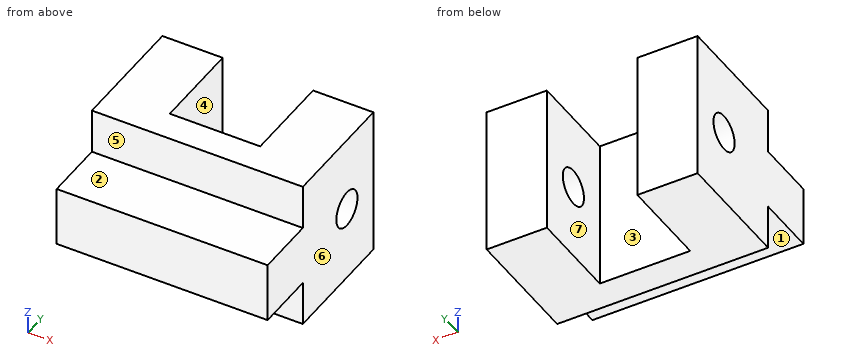
from build123d import *

# Parameters (mm, degrees)
BOSS_EXTRUDE1_DEPTH = 25
SKETCH4_R           = 3
CUT_EXTRUDE1_DEPTH  = 40
SKETCH5_W           = 35
SKETCH5_H           = 10
BOSS_EXTRUDE3_DEPTH = 10


with BuildPart() as part:
    # Sketch1 → Boss-Extrude1 (new body)
    with BuildSketch(Plane.XY):
        Polygon((0, 9.105075836), (0, -5.894924164), (-15, -5.894924164), (-15, 9.105075836), (-25, 9.105075836), (-25, -10.894924164), (10, -10.894924164), (10, 9.105075836), align=None)
    extrude(amount=-BOSS_EXTRUDE1_DEPTH)

    # Sketch4 → Cut-Extrude1 (cut)
    with BuildSketch(Plane(origin=(10, 0, 0), x_dir=(0, 0, -1), z_dir=(1, 0, 0))):
        with Locations(Location((12.5, 1.605075836, 0), (0, 0, 90))):
            Circle(SKETCH4_R)
    extrude(amount=-CUT_EXTRUDE1_DEPTH, mode=Mode.SUBTRACT)

    # Sketch5 → Boss-Extrude3 (add)
    with BuildSketch(Plane.XZ.offset(10.894924164)):
        with Locations((-7.5, -12.5)):
            Rectangle(SKETCH5_W, SKETCH5_H)
    extrude(amount=BOSS_EXTRUDE3_DEPTH)


solid = part.part
CAD build for the part. Positions are in the model's coordinates, mm. Face numbers are marked on the shaded views. A direction names the side the tool comes from. Give positions to 0.01 mm unless a question says otherwise; leave off trailing zeros. Loops run counter-clockwise (first coordinate to the right, second up) from the corner with the lowest first, then second, coordinate; pieces in that order, holes last. Notation, with made-up numbers: M -10.75,3.5 L -2.75,3.5 A18 cw -2.75,9.5 Z; hole C 50,0.5 d9. An arc over 180 degrees is marked long. Answer in a Markdown table with one row per item. Add a question column.
Item 1: Band-saw the part on A-A on y = 7. Give the cut face in (x, z), then the cut area to 3 significant figures.
Item 2: Drop flat-ended pins along their axis: P1, Ø5, axis at x = -14.5, y = -15.5, coming from the -Z side; P2, Ø11, axis at x = -4, y = -16, coming from the +Z side; P3, Ø2, axis at x = -19.5, z = -19, coming from the -Y side; P4, Ø1.5, axis at x = -10, y = -13.5, coming from the +Z side. Give the stop position or say it passes through.
Item 3: Probe probe 1 along X at (y, z) = (-5.5, -6.25); probe 2 along Z at (x, y) = (-1, -17); probe 3 along Z at (x, y) = (-18.5, 0). List the from-to ranges inside material, lowest first.
Item 4: Band-saw the part on D-D on x = -14. Give the cut face in (y, z), then the cut area to 3 significant figures.
Item 5: Mould opens along X. For the marked faces 4, 5, 6 and 7 say: +X half, -X half, draft (parallel to the pull), parting line (faces both ways), or undercut.
Item 6: Band-saw the part on B-B on x = -20.5. Give the cut face in (y, z), then the cut area to 3 significant figures.
Item 7: Tool access for the marked faces 1, 2 and 3: list every direction of +Z, -Z, +X, -X, +Y, -Y with a clear straight run to the whole face (end or side of a thin tool).
Item 8: Band-saw the part on C-C on z = -12.5. Give the cut face in (x, y), then the cut area to 3 significant figures.
Reply:
| question | item | result |
|---|---|---|
| 1 | outline | M -25,-25 L -15,-25 L -15,0 L -25,0 Z; M 0,-25 L 10,-25 L 10,0 L 0,0 Z |
| 1 | area | 500 mm^2 |
| 2 | P1 | stops at z = -17.5 |
| 2 | P2 | stops at z = 0 |
| 2 | P3 | stops at y = -10.89 |
| 2 | P4 | stops at z = -7.5 |
| 3 | probe 1 | x = -25 to -15, 0 to 10 |
| 3 | probe 2 | z = -17.5 to -7.5 |
| 3 | probe 3 | z = -25 to -15.03, -9.97 to 0 |
| 4 | outline | M -20.89,-17.5 L -10.89,-17.5 L -10.89,-25 L -5.89,-25 L -5.89,0 L -10.89,0 L -10.89,-7.5 L -20.89,-7.5 Z |
| 4 | area | 225 mm^2 |
| 5 | face 4 | undercut |
| 5 | face 5 | draft |
| 5 | face 6 | +X half |
| 5 | face 7 | undercut |
| 6 | outline | M -20.89,-17.5 L -10.89,-17.5 L -10.89,-25 L 9.11,-25 L 9.11,0 L -10.89,0 L -10.89,-7.5 L -20.89,-7.5 Z; hole C 1.61,-12.5 d6 |
| 6 | area | 572 mm^2 |
| 7 | face 1 | -Z, +X, -X, -Y |
| 7 | face 2 | +Z, +X, -X, -Y |
| 7 | face 3 | +Z, -Z, +Y |
| 8 | outline | M -25,-20.89 L 10,-20.89 L 10,-1.39 L 0,-1.39 L 0,-5.89 L -15,-5.89 L -15,-1.39 L -25,-1.39 Z; M -25,4.61 L -15,4.61 L -15,9.11 L -25,9.11 Z; M 0,4.61 L 10,4.61 L 10,9.11 L 0,9.11 Z |
| 8 | area | 705 mm^2 |
